Geometry: final body of the model. Coordinates: model frame, mm. Give positions to 0.01 mm unless a question says otherwise; leave off trailing zeros. Write each loop counter-clockwise with the first axis right and the second up, starting at its lowest first coordinate (ties: lowest second). Pieces come first, ordered by that corner, then holes. Notation, with made-up numbers: M -6,53 L -2,53 A18 cw -2,85 Z; hole C 7,72.5 d9. An arc over 180 degrees is marked long. Use one line per item in the form item = value. Start each with the question number.
Item 1: Section query C-C on y = 33.5. Return loops of the section in (x, z), then the cut area to 3 significant figures.
Item 2: Contact query for flat-ended pins moving along their axis: P1, Ø2, axis at y = 41, z = -1.5, coming from the +X side; P2, Ø4, axis at y = 17, z = 32.5, coming from the -X side; P3, Ø4, axis at y = 30, z = 33.5, coming from the -X side. Output: stop coordinate, or through.
Item 3: Material intervals for line 1 along X through (y, z) = (29, 0); line 2 along Y through (x, z) = (-54.5, -51.5), sorted ascending. Write a range as from..to.
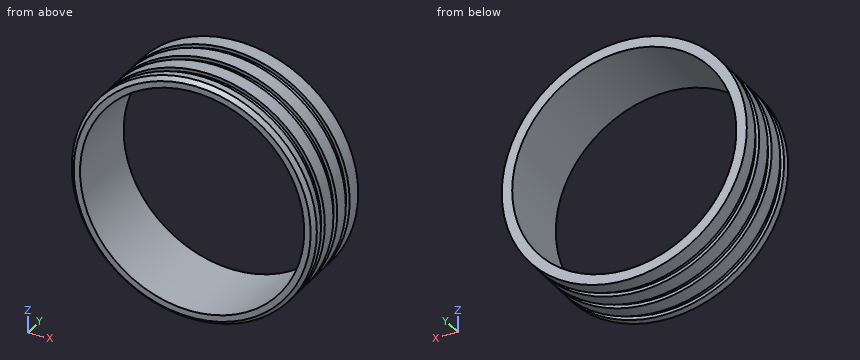
from build123d import *

# Parameters (mm, degrees)
SKETCH1_R           = 76.25
SKETCH1_R_2         = 69.75
BOSS_EXTRUDE1_DEPTH = 50.8
CHAMFER1_SIZE       = 2.5


with BuildPart() as part:
    # Sketch1 → Boss-Extrude1 (new body)
    with BuildSketch(Plane(origin=(0, 0, 0), x_dir=(1, 0, 0), z_dir=(0, 1, 0))):
        Circle(SKETCH1_R)
        Circle(SKETCH1_R_2, mode=Mode.SUBTRACT)
    extrude(amount=BOSS_EXTRUDE1_DEPTH)

    # Sketch2 → Cut-Revolve1 (revolve, cut)
    with BuildSketch(Plane.XY):
        Polygon((-76.25, 40.8), (-76.25, 36.3), (-73.75, 35.859182548), (-73.75, 41.240817452), align=None)
        Polygon((-73.75, 26.740817452), (-73.75, 21.359182548), (-76.25, 21.8), (-76.25, 26.3), align=None)
        Polygon((-73.75, 12.240817452), (-73.75, 6.859182548), (-76.25, 7.3), (-76.25, 11.8), align=None)
    revolve(axis=Axis((0, 0, 0), (0, 1, 0)), mode=Mode.SUBTRACT)

    # Chamfer1
    chamfer1_edges = [part.edges().sort_by_distance(p)[0] for p in [
        (-76.25, 0, 0),
    ]]
    chamfer(chamfer1_edges, length=CHAMFER1_SIZE)


solid = part.part
Answer sheet:
q1.outline = C 0,0 d152.5; hole C 0,0 d139.5
q1.area = 2,980 mm2
q2.P1 = 76.25
q2.P2 = -69.88
q2.P3 = -69.44
q3.line_1 = -76.25..-69.75, 69.75..76.25
q3.line_2 = 1.23..7.08, 12.02..21.58, 26.52..36.08, 41.02..50.8
